```python
from build123d import *

# Parameters (mm, degrees)
F0_W     = 180
F0_H     = 50
F1_DEPTH = 6
F2_W     = 120
F2_H     = 20
F3_DEPTH = 25
F4_R     = 19.99999


# Not quite as in the source:
# - a fillet or chamfer is up to 0.001 mm smaller than in the source, because OpenCascade refuses the exact size


with BuildPart() as f1:
    # F0 (on Right) → F1 (new body)
    with BuildSketch(Plane.YZ):
        Rectangle(F0_W, F0_H)
    extrude(amount=F1_DEPTH)

    # F2 (on face) → F3 (cut)
    with BuildSketch(Plane.YZ.offset(6)):
        with Locations((0, -15)):
            Rectangle(F2_W, F2_H)
    extrude(amount=-F3_DEPTH, mode=Mode.SUBTRACT)

    # F4 (radius 20 in the source; OpenCascade refuses exactly that, so slightly less here)
    f4_edges = [f1.edges().sort_by_distance(p)[0] for p in [
        (3, 60, -5),
        (3, -60, -5),
    ]]
    fillet(f4_edges, radius=F4_R)


solid = f1.part
```
Part model, mm, in its own coordinate system. A direction names the side the tool comes from. Round coordinates to 2 decimals unless told otherwise and drop trailing zeros. Loops run counter-clockwise (first coordinate to the right, second up) from the corner with the lowest first, then second, coordinate; pieces in that order, holes last.
1. 3-axis set-ups, long thin cutter, end or side, ignore diameter. For faces 4 (the face through (0, -1, 6)), 5 (the face through (2.958, -54.297, -11.014)): which of +Z, -Z, +X, -X, +Y, -Y reach the whole face in a straight line?
Solutions:
face 4: +Z, -Z, -X, +Y, -Y
face 5: -Z, +X, -X
2. Drill centre lines: line 1 along Z through (x, y) = (1.75, 22.5); line 2 along Y through (x, z) = (3.1, -8); line 3 along Y through (x, z) = (2.4, -9). Where is each one in solid material? Low to high.
Solutions:
line 1: z = -5 to 25
line 2: y = -90 to -50.54, 50.54 to 90
line 3: y = -90 to -52, 52 to 90
3. Slice it at C-C (y = 15). Give the cut face in (x, z).
Solutions:
outline: (0, -5) - (6, -5) - (6, 25) - (0, 25) - close
4. Slice it at B-B (y = 52). Give the cut face in (x, z).
Solutions:
outline: (0, -9) - (6, -9) - (6, 25) - (0, 25) - close
5. Two-plate mould, pull along Y, no slides. Class faces 1 (the face through (3, -90, 0)), 2 (the face through (3, 90, 0)), 3 (the face through (3, -1, -5)): pulls with the +Y half, pulls with the -Y half, needs draft (parallel to the pull), parting line crosses it, or undercut.
Solutions:
face 1: pulls with the -Y half
face 2: pulls with the +Y half
face 3: undercut
